Build history of the part. All positions in model axes, mm. A direction names the side the tool comes from. Give positions to 0.01 mm unless a question says otherwise; leave off trailing zeros. Loops run counter-clockwise (first coordinate to the right, second up) from the corner with the lowest first, then second, coordinate; pieces in that order, holes last. Notation, with made-up numbers: (85, 88) - (139, 88) arc R17 cw to (139, 96) - close; hole circle Ø4 at (50.25, -5). An arc over 180 degrees is marked (long way). Return JSON: item names as keys, results as strings. Group by question number.
1) Mould opens along X. For faces 1 (the face through (0, -14, -2)), 2 (the face through (0, -8, -5)) say: released by +X, released by -X, zero draft, split by the parting line, or undercut.
2) 3-axis set-ups, long thin cutter, end or side, ignore diameter. For faces 3 (the face through (0, -2, -99)), 4 (the face through (0, -7, 0)): which of +Z, -Z, +X, -X, +Y, -Y reach the whole face in a straight line?
3) Drop flat-ended pins along their axis: pin 1 (5 mm diameter, centred on x = 20.5, z = -66, fed in from -Y); pin 2 (6 mm diameter, centred on x = 20.5, y = -12.5, fed in from -Z). Give the stop position or say it passes through.
4) Slice it at A-A (z = -51.5). List the corners of the cut face in (x, y).
5) Drill centre lines: probe 1 along Z at (x, y) = (-8, -9); probe 2 along Z at (x, y) = (0.5, -13.25); probe 3 along Y at (x, z) = (22, -45.5). Where is each one in solid material? Low to high. Write a range as from..to.
```python
from build123d import *

# Parameters (mm, degrees)
BOSS_EXTRUDE1_DEPTH = 5
BOSS_EXTRUDE2_DEPTH = 110


with BuildPart() as part:
    # Sketch1 → Boss-Extrude1 (new body)
    with BuildSketch(Plane.XY):
        with BuildLine():
            Line((29.393876913, 0), (-29.393876913, 0))
            ThreePointArc((-29.393876913, 0), (-18.078961268, -12.607085313), (-2, -17.939338184))
            Line((-2, -17.939338184), (-2, -16))
            ThreePointArc((-2, -16), (0, -14), (2, -16))
            Line((2, -16), (2, -17.939338184))
            ThreePointArc((2, -17.939338184), (18.078961268, -12.607085313), (29.393876913, 0))
        make_face()
    extrude(amount=-BOSS_EXTRUDE1_DEPTH)

    # Sketch4 → Boss-Extrude2 (add)
    with BuildSketch(Plane(origin=(0, 0, -5), x_dir=(-1, 0, 0), z_dir=(0, 0, -1))):
        with BuildLine():
            Line((-28.284271247, -2), (28.284271247, -2))
            ThreePointArc((28.284271247, -2), (28.856406461, -1.009616054), (29.393876913, 0))
            Line((29.393876913, 0), (-29.393876913, 0))
            ThreePointArc((-29.393876913, 0), (-28.856406461, -1.009616054), (-28.284271247, -2))
        make_face()
    extrude(amount=BOSS_EXTRUDE2_DEPTH)



with BuildPart() as body_2:
    # Sketch12 → Loft4 section 0
    with BuildSketch(Plane(origin=(0, 0, -190), x_dir=(-1, 0, 0), z_dir=(0, 0, -1))):
        with BuildLine():
            Line((22.653180887, 0), (-22.653180887, 0))
            add(Edge.make_bspline(
                [(-22.653180887, 0), (-22.148977198, -1.002294604), (-21.312728642, -2.455970505), (-20.356311796, -3.834839427), (-19.691645963, -4.737243386), (-19.346258554, -5.179245011), (-17.567122979, -7.32705895), (-15.968170417, -8.864263), (-13.740314516, -10.549553496), (-13.281768803, -10.87542484), (-12.351437875, -11.495278896), (-11.878861514, -11.790005264), (-10.438884851, -12.628551852), (-9.449353735, -13.126979054), (-7.918655947, -13.779445474), (-7.400698933, -13.981090551), (-6.348352712, -14.35067626), (-5.811978486, -14.519061657), (-4.190297425, -14.964979291), (-3.100362704, -15.18241512), (-1.999999905, -15.305387205)],
                knots=[0, 0, 0, 0, 0.125, 0.1875, 0.1875, 0.25, 0.25, 0.5, 0.5, 0.5625, 0.5625, 0.625, 0.625, 0.75, 0.75, 0.8125, 0.8125, 0.875, 0.875, 1, 1, 1, 1], degree=3))
            Line((-1.999999905, -15.305387205), (-1.999999905, -13.417274226))
            add(Edge.make_bspline(
                [(2.000000095, -13.417274226), (2.000000095, -11.416233914), (9.5e-08, -11.416233914), (-1.999999905, -11.416233914), (-1.999999905, -13.417274226)],
                knots=[4.71238898, 4.71238898, 4.71238898, 6.283185307, 6.283185307, 7.853981634, 7.853981634, 7.853981634], degree=2, weights=[1, 0.707106781, 1, 0.707106781, 1]))
            Line((2.000000095, -13.417274226), (2.000000095, -15.30538728))
            add(Edge.make_bspline(
                [(2.000000095, -15.30538728), (3.11768943, -15.180478923), (4.210798102, -14.960003678), (6.358212923, -14.368193301), (7.413433781, -13.99578054), (9.48316466, -13.111567426), (10.477319809, -12.608065076), (12.391619169, -11.489443387), (13.311776359, -10.874343619), (15.080037554, -9.535479611), (15.928293309, -8.811314066), (17.550364646, -7.253254035), (18.308014434, -6.434881586), (20.428872732, -3.867681555), (21.642679013, -2.008752815), (22.653180887, 0)],
                knots=[0, 0, 0, 0, 0.125, 0.125, 0.25, 0.25, 0.375, 0.375, 0.5, 0.5, 0.625, 0.625, 0.75, 0.75, 1, 1, 1, 1], degree=3))
        make_face()
    # Sketch13 → Loft4 section 1
    with BuildSketch(Plane(origin=(0, 0, -195), x_dir=(-1, 0, 0), z_dir=(0, 0, -1))):
        with BuildLine():
            Line((22.23493812, 0), (-22.23493812, 0))
            add(Edge.make_bspline(
                [(-22.23493812, 0), (-21.740282728, -0.98514663), (-20.92074495, -2.414398694), (-19.984690863, -3.770833773), (-19.334428952, -4.658733952), (-18.995985903, -5.094588627), (-17.253288329, -7.212565885), (-15.688377335, -8.729957297), (-13.509914793, -10.396251463), (-13.061466045, -10.718755366), (-12.149963097, -11.333679684), (-11.686964176, -11.626255977), (-10.276201265, -12.459278365), (-9.306792445, -12.955267146), (-7.807228346, -13.605896686), (-7.299808046, -13.807233863), (-6.268850056, -14.176803971), (-5.743994744, -14.345317324), (-4.151377213, -14.793942329), (-3.080899423, -15.013927219), (-2.0000001, -15.139517415)],
                knots=[0, 0, 0, 0, 0.125, 0.1875, 0.1875, 0.25, 0.25, 0.5, 0.5, 0.5625, 0.5625, 0.625, 0.625, 0.75, 0.75, 0.8125, 0.8125, 0.875, 0.875, 1, 1, 1, 1], degree=3))
            Line((-2.0000001, -15.139517415), (-2.0000001, -13.255983903))
            add(Edge.make_bspline(
                [(1.9999999, -13.255983903), (1.9999999, -11.254943591), (-1e-07, -11.254943591), (-2.0000001, -11.254943591), (-2.0000001, -13.255983903)],
                knots=[1.570796327, 1.570796327, 1.570796327, 3.141592654, 3.141592654, 4.71238898, 4.71238898, 4.71238898], degree=2, weights=[1, 0.707106781, 1, 0.707106781, 1]))
            Line((1.9999999, -13.255983903), (1.9999999, -15.139517335))
            add(Edge.make_bspline(
                [(1.9999999, -15.139517335), (3.097475762, -15.012001028), (4.170492913, -14.789132022), (5.751323617, -14.342960473), (6.273417873, -14.175331497), (7.308353862, -13.804002428), (7.822701798, -13.599731703), (9.341618745, -12.939021482), (10.314473073, -12.438519778), (12.187983442, -11.328505685), (13.088646639, -10.719004096), (14.819688416, -9.393879642), (15.651226146, -8.676872801), (17.2374738, -7.139809792), (17.978680245, -6.333075632), (20.054337825, -3.803997633), (21.243421171, -1.974687006), (22.23493812, 0)],
                knots=[0, 0, 0, 0, 0.125, 0.125, 0.1875, 0.1875, 0.25, 0.25, 0.375, 0.375, 0.5, 0.5, 0.625, 0.625, 0.75, 0.75, 1, 1, 1, 1], degree=3))
        make_face()
    loft()


with BuildPart() as part_1:
    add(part.part)

    add(body_2.part)  # Loft5 merges body 2
    # Sketch15 for Loft5 → Loft5 section 0
    with BuildSketch(Plane(origin=(0, 0, -115), x_dir=(-1, 0, 0), z_dir=(0, 0, -1))):
        with BuildLine():
            Line((-28.284271247, -2), (28.284271247, -2))
            # circular arc as an exact rational Bezier (weights 1, cos(half-angle), 1)
            Bezier((28.284271247, -2), (28.873749257, -1.019237886), (29.393876913, 0), weights=[1, 0.999399358, 1])
            Line((29.393876913, 0), (-29.393876913, 0))
            Bezier((-29.393876913, 0), (-28.873749257, -1.019237886), (-28.284271247, -2), weights=[1, 0.999399358, 1])
        make_face()
    # Sketch14 → Loft5 section 1
    with BuildSketch(Plane.XY.offset(-190)):
        with BuildLine():
            Line((-21.55031948, -2), (21.549816234, -2))
            add(Edge.make_bspline(
                [(21.549816234, -2), (21.942306372, -1.348710735), (22.310082744, -0.682036694), (22.653180887, 0)],
                knots=[0.914940591, 0.914940591, 0.914940591, 0.914940591, 1, 1, 1, 1], degree=3))
            Line((22.653180887, 0), (-22.653180887, 0))
            add(Edge.make_bspline(
                [(-22.653180887, 0), (-22.309091279, -0.684007607), (-21.941428628, -1.350643187), (-21.55031948, -2)],
                knots=[0, 0, 0, 0, 0.085128394, 0.085128394, 0.085128394, 0.085128394], degree=3))
        make_face()
    loft()


solid = part_1.part
```
Results:
{
 "1": {"face 1": "undercut", "face 2": "zero draft"},
 "2": {"face 3": "+X, -X, -Y", "face 4": "+Z, +X, -X, +Y, -Y"},
 "3": {"pin 1": "y = -2", "pin 2": "z = -5"},
 "4": {"outline": "(-29.39, 0) arc R33 ccw to (-28.28, -2) - (28.28, -2) arc R33 ccw to (29.39, 0) - close"},
 "5": {"probe 1": "-195..-190, -5..0", "probe 2": "-5..0", "probe 3": "-2..0"}
}
